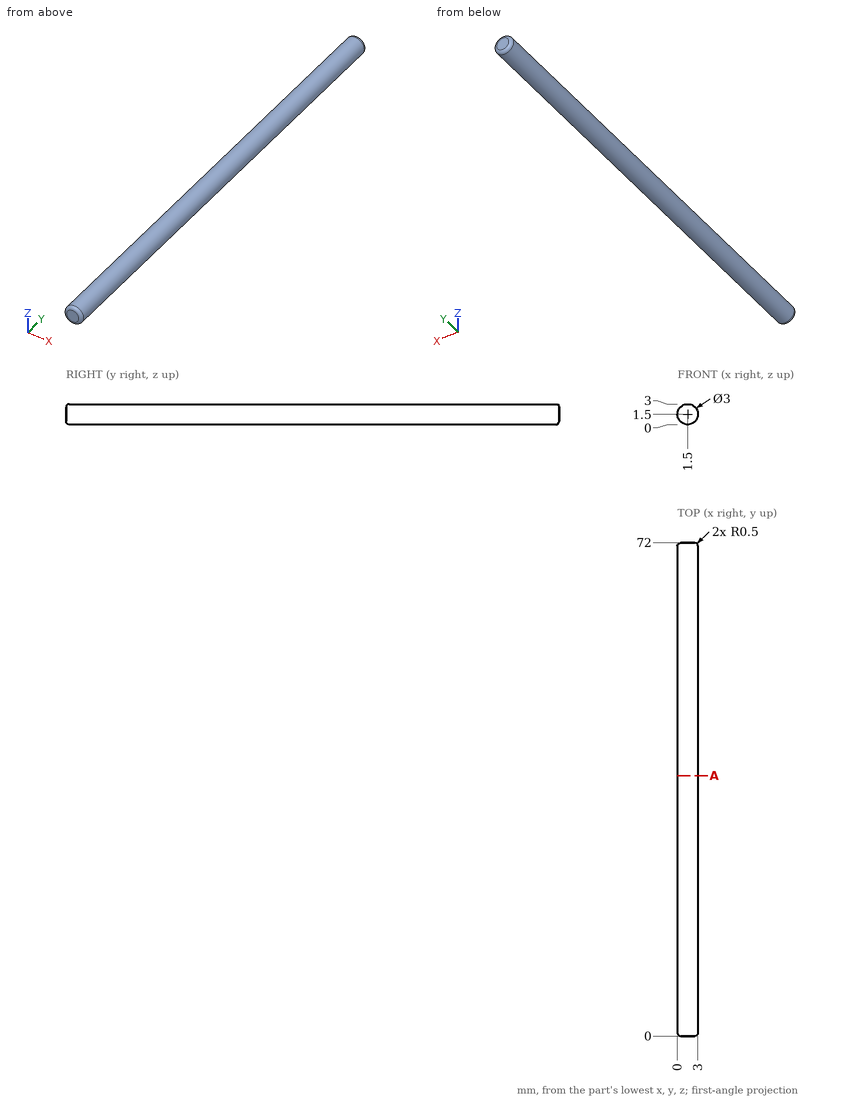
Geometry check sheet. Reference: drawing and pictorial views, mm from the part's lowest x, y, z. Round coordinates to 2 decimals unless told otherwise and drop trailing zeros. Order: outer loops, then holes, each group sorted by start corner. A loop starts at its lowest first (then second) coordinate and runs counter-clockwise, first axis right, second up. Notation, with made-up numbers: (56, 37) - (108, 37) arc R15 ccw to (108, 44) - close; hole circle Ø2 at (14, 79). An arc over 180 degrees is marked (long way). Use a Markdown table: item, result. Add a question column.
1) Section check A-A (y = 38). Record the cut outline in (x, z), then the cut area to 3 significant figures.
2) Gauge pin test, flat end, axial feed: P1, Ø1, axis at y = 14, z = 0.5, coming from the +X side. Record the tip position at first contact, or that the pin passes through.
3) Thickness scan on line 1 along Z through (x, y) = (1.6, 42.5); line 2 along Y through (x, z) = (2.6, 1.45); line 3 along X through (y, z) = (11.5, 1.3). Record the ranges inside material, lowest first.
Established:
| question | item | result |
|---|---|---|
| 1 | outline | circle Ø3 at (1.5, 1.5) |
| 1 | area | 7.07 mm2 |
| 2 | P1 | x = 2.91 |
| 3 | line 1 | 0 to 3 |
| 3 | line 2 | 0.01 to 71.99 |
| 3 | line 3 | 0.01 to 2.99 |
